from build123d import *

# Parameters (mm, degrees)
SKETCH2_R           = 8.5
SKETCH2_R_2         = 6.5
SKETCH2_R_3         = 15
SKETCH2_R_4         = 0.5
BOSS_EXTRUDE2_DEPTH = 4.5
BOSS_EXTRUDE8_START = 1.5
SKETCH2_13_R        = 6.5
SKETCH2_13_R_2      = 4
BOSS_EXTRUDE8_DEPTH = 3
SKETCH2_7_R         = 6.5
SKETCH2_7_R_2       = 4
BOSS_EXTRUDE5_DEPTH = 1.5


with BuildPart() as part:
    # Sketch2 → Boss-Extrude2 (new, symmetric)
    # profile 1 of 3: a face of its own
    with BuildSketch(Plane(origin=(-406.338605642, -287.966071976, 0), x_dir=(-0.7121905836143565, 0.7019861626920024, 0), z_dir=(0, 0, 1))):
        with BuildLine():
            ThreePointArc((-177.488840527, -503.259500631), (-177.796019748, -505.523940447), (-178.695355275, -507.624712296))
            Line((-178.695355275, -507.624712296), (-136.02252284, -496.985180209))
            Line((-136.02252284, -496.985180209), (-100.847097363, -488.214961626))
            ThreePointArc((-100.847097363, -488.214961626), (-103.513703794, -482.696139506), (-103.75016011, -476.57141291))
            Line((-103.75016011, -476.57141291), (-138.925585587, -485.341631494))
            Line((-138.925585587, -485.341631494), (-181.598418022, -495.981163581))
            ThreePointArc((-181.598418022, -495.981163581), (-178.587199112, -499.080301623), (-177.488840527, -503.259500631))
        make_face()
    # profile 2 of 3: a face of its own
    with BuildSketch(Plane(origin=(-406.338605642, -287.966071976, 0), x_dir=(-0.7121905836143565, 0.7019861626920024, 0), z_dir=(0, 0, 1))):
        with Locations((-185.988840527, -503.259500631)):
            Circle(SKETCH2_R)
        with Locations(Location((-185.988840527, -503.259500631, 0), (0, 0, 134.586572113))):
            Circle(SKETCH2_R_2, mode=Mode.SUBTRACT)
    # profile 3 of 3: a face of its own
    with BuildSketch(Plane(origin=(-406.338605642, -287.966071976, 0), x_dir=(-0.7121905836143565, 0.7019861626920024, 0), z_dir=(0, 0, 1))):
        with Locations((-88.9592679, -479.067311072)):
            Circle(SKETCH2_R_3)
        with Locations(Location((-88.9592679, -479.067311072, 0), (0, 0, 134.586572113))):
            Circle(SKETCH2_R_2, mode=Mode.SUBTRACT)
        with Locations(Location((-80.711754227, -477.010974959, 0), (0, 0, 134.586572113))):
            Circle(SKETCH2_R_4, mode=Mode.SUBTRACT)
        with Locations(Location((-97.206781573, -481.123647184, 0), (0, 0, 134.586572113))):
            Circle(SKETCH2_R_4, mode=Mode.SUBTRACT)
        with Locations(Location((-86.540048944, -488.770268334, 0), (0, 0, 134.586572113))):
            Circle(SKETCH2_R_4, mode=Mode.SUBTRACT)
        with Locations(Location((-91.378486856, -469.364353809, 0), (0, 0, 134.586572113))):
            Circle(SKETCH2_R_4, mode=Mode.SUBTRACT)
    extrude(amount=BOSS_EXTRUDE2_DEPTH, both=True)

    # Sketch2<13> → Boss-Extrude8 (add)
    with BuildSketch(Plane(origin=(-406.338605642, -287.966071976, 0), x_dir=(-0.7121905836143565, 0.7019861626920024, 0), z_dir=(0, 0, 1)).offset(BOSS_EXTRUDE8_START)):
        with Locations(Location((-88.9592679, -479.067311072, 0), (0, 0, 134.586572113))):
            Circle(SKETCH2_13_R)
        with Locations(Location((-88.9592679, -479.067311072, 0), (0, 0, 134.586572113))):
            Circle(SKETCH2_13_R_2, mode=Mode.SUBTRACT)
    extrude(amount=BOSS_EXTRUDE8_DEPTH)

    # Sketch2<7> → Boss-Extrude5 (add, symmetric)
    with BuildSketch(Plane(origin=(-406.338605642, -287.966071976, 0), x_dir=(-0.7121905836143565, 0.7019861626920024, 0), z_dir=(0, 0, 1))):
        with Locations(Location((-185.988840527, -503.259500631, 0), (0, 0, 134.586572113))):
            Circle(SKETCH2_7_R)
        with Locations(Location((-185.988840527, -503.259500631, 0), (0, 0, 134.586572113))):
            Circle(SKETCH2_7_R_2, mode=Mode.SUBTRACT)
    extrude(amount=BOSS_EXTRUDE5_DEPTH, both=True)


solid = part.part
Work out the finished part from the listing and answer in its coordinate system (mm). A direction names the side the tool comes from. Give positions to 0.01 mm unless a question says otherwise; leave off trailing zeros. Write each loop counter-clockwise with the first axis right and the second up, starting at its lowest first coordinate (ties: lowest second). Pieces come first, ordered by that corner, then holes. Notation, with made-up numbers: M 40,31.5 L 90,31.5 A9 ccw 90,38.5 Z; hole C 14.5,25.5 d6. An arc over 180 degrees is marked long. Answer as CSV lines item,"result".
Q1. A tool of negligible diameter and unlimited length cuts with its end or side. For faces 5 (the cylindrical face through (73.635, -63.11, 2.979)), 6 (the flat face through (-11, -9, 1.5)), 7 (the cylindrical face through (-3.311, -11.377, 2.979)), from which of +Z, -Z, +X, -X, +Y, -Y can it reach the whole face along a straight path? Write none if from no direction.
A:
face 5,"+Z"
face 6,"-Z"
face 7,"+Z, -Z"
Q2. A cutting plane is placed at D-D on y = 1. Write down the section's boundary in (x, z).
A:
outline,"M -17.66,-4.5 L 4.29,-4.5 L 4.29,4.5 L -17.66,4.5 Z"
Q3. Given P1, Ø10.5, axis at x = 79.4, y = -60.11, coming from the +Z side; P2, Ø4, axis at y = -21, z = -1.5, coming from the -X side; P3, Ø3, axis at y = -30.5, z = -0.5, coming from the +X side; P4, Ø5, axis at x = -6.68, y = -9.23, coming from the +Z side, each flat-ended and moving along its own axis, determine where each tip first touches the part or whether it passes through.
A:
P1,"stops at z = 1.5"
P2,"stops at x = -18.06"
P3,"stops at x = 43.64"
P4,"passes through"
Q4. A cutting plane is placed at C-C on x = 67. Write down the section's boundary in (y, z), plus the area to 3 significant figures.
A:
outline,"M -59.75,-4.5 L -45.81,-4.5 L -45.81,4.5 L -59.75,4.5 Z"
area,"125 mm²"
Q5. A cutting plane is placed at A-A on y = -60. Write down the section's boundary in (x, z).
A:
outline,"M 67.42,-4.5 L 72.9,-4.5 L 72.9,-1.5 L 75.4,-1.5 L 75.4,1.5 L 72.9,1.5 L 72.9,4.5 L 67.42,4.5 Z; M 83.4,-1.5 L 85.9,-1.5 L 85.9,-4.5 L 87.9,-4.5 L 87.9,4.5 L 85.9,4.5 L 85.9,1.5 L 83.4,1.5 Z"
Q6. A cutting plane is placed at B-B on z = -2.75. Write down the section's boundary in (x, y).
A:
outline,"M 2.1,-21.39 L 71.17,-62.21 A8.5 ccw long 77.27,-51.88 L 8.2,-11.06 A15 ccw long Z; hole C -14,-4.9 d1; hole C -6.68,-9.23 d13; hole C -11.77,-17.84 d1; hole C -1.6,-0.62 d1; hole C 0.63,-13.55 d1; hole C 79.4,-60.11 d13"
Q7. Find the intervals of material crossed by probe 1 along Y at (x, z) = (79, 0.75); probe 2 along Y at (x, z) = (-14, -0.25); probe 3 along X at (y, z) = (-9.5, 3.25), in increasing order. Write a range as [from, to].
A:
probe 1,"y = [-68.6, -64.09], [-56.13, -51.62]"
probe 2,"y = [-22.32, -5.4], [-4.4, 3.87]"
probe 3,"x = [-21.68, -10.67], [-2.69, 8.31]"
Q8. The mould has two halves that part along Y. Classify faces 1 (the cylindrical face through (73.635, -63.11, -3.021)), 2 (the flat face through (25, -26, 4.5)), 3 (the flat face through (75, -60, -1.5)), 4 (the cylindrical face through (86.57, -64.68, -0.06)): +Y half, -Y half, draft (parallel to the pull), parting line (faces both ways), or undercut.
A:
face 1,"undercut"
face 2,"draft"
face 3,"undercut"
face 4,"parting line"
